Autodesk Inventor part; units mm, degrees
ref_plane "YZ Plane" through (0, 0, 0) normal (1, 0, 0) x (0, 1, 0)
ref_plane "XZ Plane" through (0, 0, 0) normal (0, 1, 0) x (-1, 0, 0)
ref_plane "XY Plane" through (0, 0, 0) normal (0, 0, 1) x (1, 0, 0)
sketch "Sketch1" plane through (0, 0, 0) normal (0, 1, 0) x (-1, 0, 0)
  line L0 (0, 0) -> (-63, 0)
  line L1 (-63, 0) -> (-63, -74)
  line L2 (-63, -74) -> (0, -74)
  line L3 (0, -74) -> (0, 0)
  dimension "d0" = 63
  dimension "d1" = 74
extrude "Extrusion1" add sketch "Sketch1" along normal blind 2
sketch "Sketch2" plane through (0, 2, 0) normal (0, 1, 0) x (1, 0, 0)
  circle A0 centre (59, 8) radius 1
  line L0 (0, 0) -> (63, 0)
  line L1 (63, 0) -> (63, 74)
  circle A1 centre (10, 59) radius 1
  line L2 (63, 74) -> (0, 74)
  line L3 (0, 74) -> (0, 0)
  dimension "d4" = 2
  dimension "d5" = 8
  dimension "d6" = 4
  dimension "d7" = 2
  dimension "d8" = 15
  dimension "d9" = 10
extrude "Extrusion2" cut sketch "Sketch2" against normal up to next contours A0 | A1
sketch "Sketch3" plane through (0, 0, 0) normal (0, -1, 0) x (1, 0, 0)
  line L0 (2.25, -2.25) -> (60.75, -2.25)
  line L1 (60.75, -2.25) -> (60.75, -71.75)
  line L2 (60.75, -71.75) -> (2.25, -71.75)
  line L3 (2.25, -71.75) -> (2.25, -2.25)
  line L4 (0, 0) -> (63, 0)
  line L5 (0, -74) -> (0, 0)
  line L6 (3.25, -3.25) -> (59.75, -3.25)
  line L7 (59.75, -3.25) -> (59.75, -70.75)
  line L8 (59.75, -70.75) -> (3.25, -70.75)
  line L9 (3.25, -70.75) -> (3.25, -3.25)
  dimension "d12" = 58.5
  dimension "d13" = 69.5
  dimension "d14" = 2.25
  dimension "d15" = 2.25
  dimension "d16" = 56.5
  dimension "d17" = 67.5
  dimension "d18" = 1
  dimension "d19" = 1
extrude "Extrusion3" add sketch "Sketch3" along normal blind 1
chamfer "Chamfer1" distance 1 angle 45 1 edges at (3.25, -1, -37) measured on face at (3.25, -0.3333, -48.25)
chamfer "Chamfer2" distance 1 angle 45 1 edges at (31.5, -1, -3.25) measured on face at (40.9167, -0.3335, -3.25)
chamfer "Chamfer3" distance 1 angle 45 1 edges at (59.75, -1, -37) measured on face at (59.75, -0.6667, -27.5538)
chamfer "Chamfer4" distance 1 angle 45 1 edges at (31.5, -1, -70.75) measured on face at (22.0833, -0.6668, -70.75)
sketch "Sketch4" plane through (0, 2, 0) normal (0, 1, 0) x (1, 0, 0)
  circle A0 centre (4.5, 69.5) radius 1.75
  line L0 (63, 74) -> (0, 74)
  line L1 (0, 74) -> (0, 0)
  circle A1 centre (58.5, 69.5) radius 1.75
  line L2 (63, 0) -> (63, 74)
  circle A2 centre (58.5, 4.5) radius 1.75
  line L3 (0, 0) -> (63, 0)
  dimension "d34" = 3.5
  dimension "d35" = 4.5
  dimension "d36" = 4.5
  dimension "d37" = 3.5
  dimension "d38" = 4.5
  dimension "d39" = 4.5
  dimension "d40" = 3.5
  dimension "d41" = 4.5
  dimension "d42" = 4.5
extrude "Extrusion4" cut sketch "Sketch4" against normal up to next contours A0 | A1 | A2
properties part number "top"
Source: CAD feature listing. Evaluate the final solid. Frame: model axes, mm. A direction names the side the tool comes from. Round coordinates to 2 decimals unless told otherwise and drop trailing zeros. Use a Markdown table: item, result. Add a question column.
1. Line query: probe 1 along X at (y, z) = (1.55, -69.5); probe 2 along Z at (x, y) = (10, 0.75); probe 3 along X at (y, z) = (0.6, -8). Output: solid intervals per line, ascending.
2. Section query C-C (z = -69.5). Give the number of separate pieces and of enclosed holes in the cut face, then the cut area to 3 significant figures.
3. Set-up query: faces 5 (the flat face through (32, 0, -37)), 6 (the cylindrical face through (58, 1, -8)), 7 (the flat face through (0, 1, -38)). Return all of +Z, -Z, +X, -X, +Y, -Y with unobstructed straight access to the full face (end or side cutting, diameter ignored); none if empty.
4. First-contact query: pin 1 (4 mm diameter, centred on x = 44.5, z = -55, fed in from -Y). Flat tip, straight axial feed; report the tip coordinate or a pass-through.
5. Mould query, pull axis Z, two halves, no side actions, for faces 1 (the cylindrical face through (60.117, 1.045, -3.83)), 2 (the flat face through (63, 1, -36)), 3 (the flat face through (31, 1, 0)), 4 (the flat face through (32, 1, -74)). Classes: +Z half, -Z half, draft (parallel to the pull), parting line (faces both ways), or undercut.
Derived:
| question | item | result |
|---|---|---|
| 1 | probe 1 | 0 to 2.75, 6.25 to 56.75, 60.25 to 63 |
| 1 | probe 2 | -74 to -60, -58 to 0 |
| 1 | probe 3 | 0 to 58, 60 to 63 |
| 2 | separate pieces | 3 |
| 2 | enclosed holes | 0 |
| 2 | area | 113 mm2 |
| 3 | face 5 | -Y |
| 3 | face 6 | +Y |
| 3 | face 7 | +Z, -Z, -X, +Y, -Y |
| 4 | pin 1 | y = 0 |
| 5 | face 1 | undercut |
| 5 | face 2 | draft |
| 5 | face 3 | +Z half |
| 5 | face 4 | -Z half |
